The listing builds one solid part. Answer for the finished solid, in the listing's coordinates (mm). Give positions to 0.01 mm unless a question says otherwise; leave off trailing zeros. Order: outer loops, then holes, each group sorted by start corner. A loop starts at its lowest first (then second) coordinate and runs counter-clockwise, first axis right, second up. Notation, with made-up numbers: (64, 83.5) - (102, 83.5) arc R22 cw to (102, 121.5) - close; hole circle Ø3 at (87.25, 20). An arc over 180 degrees is marked (long way). Answer in a Markdown table with one row per item.
from build123d import *

# Parameters (mm, degrees)
F0_W     = 849.2
F0_H     = 450
F1_DEPTH = 25.4


with BuildPart() as f1:
    # F0 (on Front) → F1 (new body)
    with BuildSketch(Plane.XZ):
        Polygon((0, 2427), (0, 0), (25.4, 0), (25.4, 500), (874.6, 500), (874.6, 0), (900, 0), (900, 2427), align=None)
        with Locations((450, 750.4)):
            Rectangle(F0_W, F0_H, mode=Mode.SUBTRACT)
        with Locations((450, 1225.8)):
            Rectangle(F0_W, F0_H, mode=Mode.SUBTRACT)
        with Locations((450, 1701.2)):
            Rectangle(F0_W, F0_H, mode=Mode.SUBTRACT)
        with Locations((450, 2176.6)):
            Rectangle(F0_W, F0_H, mode=Mode.SUBTRACT)
    extrude(amount=F1_DEPTH)


solid = f1.part
Item 1: Consider line 1 (Z direction, x = 265.5, y = -16.5); line 2 (X direction, y = -12.5, z = 702.5). Determine where each line is inside the solid, lowest interval first.
Answer block:
| item | result |
|---|---|
| line 1 | 500 to 525.4, 975.4 to 1000.8, 1450.8 to 1476.2, 1926.2 to 1951.6, 2401.6 to 2427 |
| line 2 | 0 to 25.4, 874.6 to 900 |
Item 2: This flat-tipped pin is pushed along its axis until it touches: P1, Ø4, axis at x = 160, y = -22.5, coming from the -Z side. Where does it stop, or does it pass through?
Answer block:
| item | result |
|---|---|
| P1 | z = 500 |
Item 3: Find section B-B on x = 81. Write down the section's boundary in (y, z).
Answer block:
| item | result |
|---|---|
| outline | (-25.4, 500) - (0, 500) - (0, 525.4) - (-25.4, 525.4) - close; (-25.4, 975.4) - (0, 975.4) - (0, 1000.8) - (-25.4, 1000.8) - close; (-25.4, 1450.8) - (0, 1450.8) - (0, 1476.2) - (-25.4, 1476.2) - close; (-25.4, 1926.2) - (0, 1926.2) - (0, 1951.6) - (-25.4, 1951.6) - close; (-25.4, 2401.6) - (0, 2401.6) - (0, 2427) - (-25.4, 2427) - close |
Item 4: Find section C-C on y = -16. Write down the section's boundary in (x, z).
Answer block:
| item | result |
|---|---|
| outline | (0, 0) - (25.4, 0) - (25.4, 500) - (874.6, 500) - (874.6, 0) - (900, 0) - (900, 2427) - (0, 2427) - close; hole (25.4, 525.4) - (874.6, 525.4) - (874.6, 975.4) - (25.4, 975.4) - close; hole (25.4, 1000.8) - (874.6, 1000.8) - (874.6, 1450.8) - (25.4, 1450.8) - close; hole (25.4, 1476.2) - (874.6, 1476.2) - (874.6, 1926.2) - (25.4, 1926.2) - close; hole (25.4, 1951.6) - (874.6, 1951.6) - (874.6, 2401.6) - (25.4, 2401.6) - close |
Item 5: Find section A-A on z = 2185.5. Write down the section's boundary in (x, y), then the cut area to 3 significant figures.
Answer block:
| item | result |
|---|---|
| outline | (0, -25.4) - (25.4, -25.4) - (25.4, 0) - (0, 0) - close; (874.6, -25.4) - (900, -25.4) - (900, 0) - (874.6, 0) - close |
| area | 1,290 mm² |
